```python
from build123d import *

# Parameters (mm, degrees)
BOSS_EXTRUDE1_DEPTH = 1.6
BOSS_EXTRUDE2_DEPTH = 1.6
BOSS_EXTRUDE3_DEPTH = 3.3
BOSS_EXTRUDE4_DEPTH = 1
BOSS_EXTRUDE5_DEPTH = 6.8
SKETCH7_W           = 1.5
SKETCH7_H           = 1.538953592
BOSS_EXTRUDE6_DEPTH = 4.18
SKETCH8_R           = 1
BOSS_EXTRUDE7_DEPTH = 0.8
SKETCH9_W           = 5
SKETCH9_H           = 1.7
CUT_EXTRUDE1_DEPTH  = 8.09
BOSS_EXTRUDE8_DEPTH = 4
SKETCH12_R          = 0.23
BOSS_EXTRUDE9_DEPTH = 3


with BuildPart() as part:
    # Sketch1 → Boss-Extrude1 (new body)
    with BuildSketch(Plane(origin=(0, 0, 0), x_dir=(1, 0, 0), z_dir=(0, 1, 0))):
        with BuildLine():
            Line((9.7, 0), (9.7, 0.989309127))
            ThreePointArc((9.7, 0.989309127), (10.261810116, 0.507786079), (10.8, 0))
            Line((10.8, 0), (10.8, -2.69))
            Line((10.8, -2.69), (6.8, -2.69))
            Line((6.8, -2.69), (6.8, 2.861046408))
            ThreePointArc((6.8, 2.861046408), (7.458731009, 2.513392708), (8.1, 2.134494679))
            Line((8.1, 2.134494679), (8.1, 0))
            ThreePointArc((8.1, 0), (8.9, -0.8), (9.7, 0))
        make_face()
    extrude(amount=BOSS_EXTRUDE1_DEPTH)

    # Sketch2 → Boss-Extrude2 (add)
    with BuildSketch(Plane(origin=(0, 1.6, 0), x_dir=(1, 0, 0), z_dir=(0, 1, 0))):
        with BuildLine():
            Line((6.8, -2.69), (6.8, 2.861046408))
            ThreePointArc((6.8, 2.861046408), (5.814434387, 3.309058403), (4.8, 3.687181666))
            Line((4.8, 3.687181666), (4.8, -2.69))
            Line((4.8, -2.69), (6.8, -2.69))
        make_face()
    extrude(amount=-BOSS_EXTRUDE2_DEPTH)

    # Sketch3 → Boss-Extrude3 (add)
    with BuildSketch(Plane(origin=(0, 1.6, 0), x_dir=(1, 0, 0), z_dir=(0, 1, 0))):
        with BuildLine():
            Line((6.8, -2.69), (6.8, 2.861046408))
            ThreePointArc((6.8, 2.861046408), (4.219046242, 3.868311453), (1.5, 4.4))
            Line((1.5, 4.4), (1.5, 1.9))
            Line((1.5, 1.9), (0, 1.9))
            Line((0, 1.9), (0, -2.69))
            Line((0, -2.69), (6.8, -2.69))
        make_face()
    extrude(amount=BOSS_EXTRUDE3_DEPTH)

    # Sketch4 → Boss-Extrude4 (add)
    with BuildSketch(Plane.XY.offset(2.69)):
        Polygon((6.8, 1.6), (6.8, 0), (4.8, 0), (4.8, 1.6), (0, 1.6), (0, 4.9), (6.8, 4.9), align=None)
    extrude(amount=BOSS_EXTRUDE4_DEPTH)

    # Sketch6 → Boss-Extrude5 (add)
    with BuildSketch(Plane(origin=(6.8, 0, 0), x_dir=(0, 0, -1), z_dir=(1, 0, 0))):
        with BuildLine():
            Line((-2.69, 9.08), (2.861046408, 9.08))
            Line((2.861046408, 9.08), (2.861046408, 4.9))
            Line((2.861046408, 4.9), (1.85, 4.9))
            ThreePointArc((1.85, 4.9), (2.74, 5.79), (1.85, 6.68))
            Line((1.85, 6.68), (-2.69, 6.68))
            Line((-2.69, 6.68), (-2.69, 9.08))
        make_face()
    extrude(amount=-BOSS_EXTRUDE5_DEPTH)

    # Sketch7 → Boss-Extrude6 (add)
    with BuildSketch(Plane(origin=(0, 4.9, 0), x_dir=(1, 0, 0), z_dir=(0, 1, 0))):
        with Locations((0.75, 3.630523204)):
            Rectangle(SKETCH7_W, SKETCH7_H)
        with BuildLine():
            Line((1.5, 4.4), (1.5, 2.861046408))
            Line((1.5, 2.861046408), (6.8, 2.861046408))
            ThreePointArc((6.8, 2.861046408), (4.219046242, 3.868311453), (1.5, 4.4))
        make_face()
    extrude(amount=BOSS_EXTRUDE6_DEPTH)

    # Sketch8 → Boss-Extrude7 (add)
    with BuildSketch(Plane.XZ):
        with Locations((6.3, 0)):
            Circle(SKETCH8_R)
    extrude(amount=BOSS_EXTRUDE7_DEPTH)

    # Sketch9 → Cut-Extrude1 (cut, through all)
    with BuildSketch(Plane.XY.offset(2.69)):
        with Locations((2.5, 8.23)):
            Rectangle(SKETCH9_W, SKETCH9_H)
    extrude(amount=-CUT_EXTRUDE1_DEPTH, mode=Mode.SUBTRACT)

    # Mirror3: part across plane


with BuildPart() as part_1:
    add(part.part)
    add(part.part.mirror(Plane(origin=(0, 4.9, -1.9), x_dir=(0, 0, 1), z_dir=(1, 0, 0))))

    # Sketch10 → Boss-Extrude8 (add, symmetric)
    with BuildSketch(Plane(origin=(0, 0, 0), x_dir=(0, 0, -1), z_dir=(1, 0, 0))):
        Polygon((0, 7.38), (-5.3, 7.38), (-5.3, 10.6), (-2.6, 10.6), (-2.6, 8.08), (0, 8.08), (2.7, 8.08), (2.7, 7.38), align=None)
    extrude(amount=BOSS_EXTRUDE8_DEPTH, both=True)

    # Sketch12 → Boss-Extrude9 (add)
    with BuildSketch(Plane(origin=(0, 10.6, 0), x_dir=(1, 0, 0), z_dir=(0, 1, 0))):
        with Locations((0, -3.92)):
            Circle(SKETCH12_R)
        with Locations((1.27, -3.92)):
            Circle(SKETCH12_R)
        with Locations((2.54, -3.92)):
            Circle(SKETCH12_R)
        with Locations((-1.27, -3.92)):
            Circle(SKETCH12_R)
        with Locations((-2.54, -3.92)):
            Circle(SKETCH12_R)
    extrude(amount=BOSS_EXTRUDE9_DEPTH)


solid = part_1.part
```
Verification items for the finished model (mm, model axes). A direction names the side the tool comes from. Give positions to 0.01 mm unless a question says otherwise; leave off trailing zeros. Order: outer loops, then holes, each group sorted by start corner. A loop starts at its lowest first (then second) coordinate and runs counter-clockwise, first axis right, second up. Notation, with made-up numbers: M -34.5,-3 L -3.5,-3 A19 cw -3.5,16 Z; hole C 32,52.5 d10. An arc over 180 degrees is marked long. Return JSON: item names as keys, results as strings. Group by question number.
1) Section check B-B on z = 1.25. Record the cut outline in (x, y), and give its area (3 significant figures).
2) Section check C-C on x = 0. Record the cut outline in (y, z).
3) Go/stop test with flat-tipped pins: pin 1 Ø0.5 at (y, z) = (8.5, 0) entering from -X; pin 2 Ø6 at (x, y) = (5, 10.5) entering from +Z; pin 3 Ø5 at (y, z) = (8, 1.5) entering from +X; pin 4 Ø1.3 at (x, z) = (2, 4.5) entering from -Y. Record where each tip stops, or that it passes through.
4) Access from +Z, -Z, +X, -X, +Y, -Y to the whole of each face (thin tool, end or side, straight path). Record for faces 1 (the face through (9, 1, 2.69)), 2 (the face through (8, 1.6, 1)), 3 (the face through (1.5, 3, -3)), 4 (the face through (-9.7, 0.8, -0.5)).
5) Section check D-D on y = 7. Record the cut outline in (x, z), and give its area (3 significant figures).
6) Scan lines: line 1 (Y direction, x = 3.5, z = -1.75); line 2 (X direction, y = 0.75, z = 2.5); line 3 (Y direction, x = 3.75, z = 3). Record each from-to range of solid material in increasing order.
7) Section check A-A on y = 0.25. Record the cut outline in (x, z), and give its area (3 significant figures).
8) Mould release check, pull along X, two halves, no side actions. Record for faces 5 (the face through (10.254, 0.789, -0.515)), 6 (the face through (0, 9, 5.3)), 7 (the face through (0, 1.6, 0)): pulls with the +X half, pulls with the -X half, needs draft (parallel to the pull), parting line crosses it, or undercut.
Answer block:
{
 "1": {"outline": "M -10.8,0 L -4.8,0 L -4.8,1.6 L 4.8,1.6 L 4.8,0 L 10.8,0 L 10.8,1.6 L 6.8,1.6 L 6.8,4.9 L -6.8,4.9 L -6.8,1.6 L -10.8,1.6 Z; M -6.8,6.68 L 6.8,6.68 L 6.8,9.08 L 5,9.08 L 5,7.38 L 4,7.38 L 4,8.08 L -4,8.08 L -4,7.38 L -5,7.38 L -5,9.08 L -6.8,9.08 Z", "area": "85.3 mm^2"},
 "2": {"outline": "M 1.6,-1.9 L 4.9,-1.9 L 4.9,-4.4 L 7.38,-4.4 L 7.38,-2.7 L 8.08,-2.7 L 8.08,2.6 L 10.6,2.6 L 10.6,3.69 L 13.6,3.69 L 13.6,4.15 L 10.6,4.15 L 10.6,5.3 L 7.38,5.3 L 7.38,2.69 L 6.68,2.69 L 6.68,-1.85 A0.89 cw 4.9,-1.85 L 4.9,3.69 L 1.6,3.69 Z"},
 "3": {"pin 1": "stops at x = -6.8", "pin 2": "stops at z = 5.3", "pin 3": "stops at x = 6.8", "pin 4": "stops at y = 7.38"},
 "4": {"face 1": "+Z, +X, +Y, -Y", "face 2": "+Z, -Z, +X, +Y", "face 3": "-Z, -Y", "face 4": "-Z, +Y, -Y"},
 "5": {"outline": "M -6.8,-2.86 A15.5 ccw -1.5,-4.4 L 1.5,-4.4 A15.5 ccw 6.8,-2.86 L 6.8,2.69 L -6.8,2.69 Z", "area": "90.1 mm^2"},
 "6": {"line 1": "y = 1.6 to 4.9, 6.68 to 8.08", "line 2": "x = -10.8 to -4.8, 4.8 to 10.8", "line 3": "y = 1.6 to 4.9, 7.38 to 10.6"},
 "7": {"outline": "M -10.8,0 A15.5 ccw -9.7,-0.99 L -9.7,0 A0.8 cw -8.1,0 L -8.1,-2.13 A15.5 ccw -4.8,-3.69 L -4.8,3.69 L -6.8,3.69 L -6.8,2.69 L -10.8,2.69 Z; M 4.8,-3.69 A15.5 ccw 8.1,-2.13 L 8.1,0 A0.8 cw 9.7,0 L 9.7,-0.99 A15.5 ccw 10.8,0 L 10.8,2.69 L 6.8,2.69 L 6.8,3.69 L 4.8,3.69 Z", "area": "55.1 mm^2"},
 "8": {"face 5": "pulls with the +X half", "face 6": "needs draft", "face 7": "undercut"}
}
